Geometry: see drawing. Coordinates: mm, zero at the bounding-box minimum. Coordinates: 2 decimals unless noted, no trailing zeros. Order: outer loops, then holes, each group sorted by start corner. A loop starts at its lowest first (then second) coordinate and runs counter-clockwise, first axis right, second up.
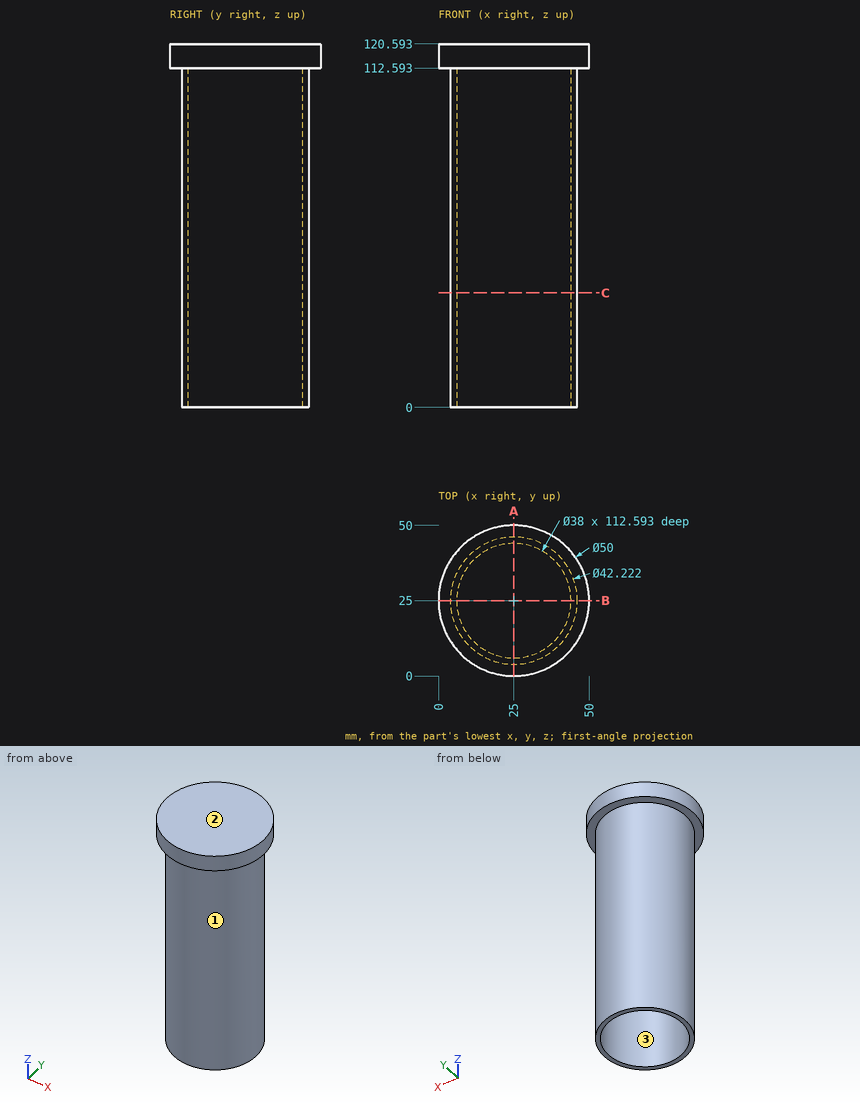
Q1. Pull-direction query (X, two-part tool) for the marked faces 1, 2 and 3; classes: pulls with the +X half, pulls with the -X half, needs draft (parallel to the pull), parting line crosses it, or undercut.
Solutions:
face 1: parting line crosses it
face 2: needs draft
face 3: undercut
Q2. Material intervals for line 1 along Y through (x, z) = (25, 23.5); line 2 along Z through (x, y) = (16, 20); line 3 along Y through (x, z) = (28.5, 11.5) (1 decimal), sorted ascending.
Solutions:
line 1: y = 3.89 to 6, 44 to 46.11
line 2: z = 112.59 to 120.59
line 3: y = 4.2 to 6.3, 43.7 to 45.8
Q3. Section query A-A on x = 25. Output: boundary loops of the cut face in (y, z).
Solutions:
outline: (0, 112.59) - (3.89, 112.59) - (3.89, 0) - (6, 0) - (6, 112.59) - (44, 112.59) - (44, 0) - (46.11, 0) - (46.11, 112.59) - (50, 112.59) - (50, 120.59) - (0, 120.59) - close
Q4. Pin query (flat end, axial travel): P1, Ø1.5, axis at y = 27, z = 36, coming from the -X side; P2, Ø15, axis at x = 27, y = 20.5, coming from the -Z side; P3, Ø2, axis at y = 15, z = 63.5, coming from the -X side. Return the tip coordinate at first contact, or that it passes through.
Solutions:
P1: stops at x = 3.93
P2: stops at z = 112.59
P3: stops at x = 5.9
Q5. Section query C-C on z = 38. Output: boundary loops of the cut face in (x, y).
Solutions:
outline: circle Ø42.22 at (25, 25); hole circle Ø38 at (25, 25)
